Work out the finished part from the listing and answer in its coordinate system (mm). A direction names the side the tool comes from. Give positions to 0.01 mm unless a question says otherwise; leave off trailing zeros. Order: outer loops, then holes, each group sorted by start corner. A loop starts at its lowest first (then second) coordinate and runs counter-clockwise, first axis right, second up. Notation, with made-up numbers: (9, 66.25) - (50, 66.25) arc R23 ccw to (50, 85.25) - close; hole circle Ø11 at (-13, 65.5). An arc over 180 degrees is marked (long way). Put each result on its own line as item: value.
```python
from build123d import *

# Parameters (mm, degrees)
SZKIC1_R                    = 42
DODANIE_WYCI_GNI_CIE1_DEPTH = 200
SFAZOWANIE1_SIZE            = 10
SKORUPA1_T                  = -0.2
SZKIC8_R                    = 32
DODANIE_WYCI_GNI_CIE4_DEPTH = 0.2


with BuildPart() as part:
    # Szkic1 → Dodanie-wyciągnięcie1 (new body)
    with BuildSketch(Plane(origin=(0, 0, 0), x_dir=(1, 0, 0), z_dir=(0, 1, 0))):
        with Locations(Location((0, 0, 0), (0, 0, 270))):
            Circle(SZKIC1_R)
    extrude(amount=DODANIE_WYCI_GNI_CIE1_DEPTH)

    # Sfazowanie1
    sfazowanie1_edges = [part.edges().sort_by_distance(p)[0] for p in [
        (0, 0, -42),
        (0, 200, -42),
    ]]
    chamfer(sfazowanie1_edges, length=SFAZOWANIE1_SIZE)

    # Skorupa1
    skorupa1_openings = [part.faces().sort_by_distance(p)[0] for p in [
        (0, 200, 0),
    ]]
    offset(amount=SKORUPA1_T, openings=skorupa1_openings, kind=Kind.INTERSECTION)

    # Szkic8 → Dodanie-wyciągnięcie4 (add)
    with BuildSketch(Plane(origin=(0, 200, 0), x_dir=(1, 0, 0), z_dir=(0, 1, 0))):
        Circle(SZKIC8_R)
    extrude(amount=-DODANIE_WYCI_GNI_CIE4_DEPTH)


solid = part.part
```
(1) Determine the mould class of faces 1 (the face through (9.76, 199.51, 30.99)), 2 (the face through (-19.71, 0.68, -25.71)), 3 (the face through (0, 199.8, 0)), 4 (the face through (12.62, 98.74, 40.06)) for opening direction Y: pulls with the +Y half, pulls with the -Y half, needs draft (parallel to the pull), parting line crosses it, or undercut.
Geometry check:
face 1: pulls with the +Y half
face 2: undercut
face 3: undercut
face 4: needs draft
(2) A tool of negligible diameter and unlimited length cuts with its end or side. For faces 5 (the face through (9.76, 0.49, 30.99)), 6 (the face through (12.56, 98.74, 39.87)), from which of +Z, -Z, +X, -X, +Y, -Y can it reach the whole face along a straight path? Write none if from no direction.
Geometry check:
face 5: -Y
face 6: none
(3) Straight lines are drawn through the part: line 1 (Y direction, x = 17, z = 14.5); line 2 (X direction, y = 144, z = 0); line 3 (X direction, y = 107, z = -29). For each, find the intervals that lie inside material, in ascending order.
Geometry check:
line 1: y = 0 to 0.2, 199.8 to 200
line 2: x = -42 to -41.8, 41.8 to 42
line 3: x = -30.38 to -30.1, 30.1 to 30.38
(4) Given pin 1 (10 mm diameter, centred on y = 122.5, z = -25.5, fed in from -X); pin 2 (6 mm diameter, centred on y = 68, z = 11.5, fed in from +X); pin 3 (1 mm diameter, centred on y = 178, z = -12, fed in from +X), each flat-ended and moving along its own axis, determine where each tip first touches the part or whether it passes through.
Geometry check:
pin 1: stops at x = -36.66
pin 2: stops at x = 41.13
pin 3: stops at x = 40.39
(5) Section C-C, the plane y = 171.5 is taken. Write down the section's boundary in (x, z).
Geometry check:
outline: circle Ø84 at (0, 0); hole circle Ø83.6 at (0, 0)
(6) Section B-B, the plane x = 0 is taken. Write down the section's boundary in (y, z), then the cut area to 3 significant figures.
Geometry check:
outline: (0, -32) - (10, -42) - (190, -42) - (200, -32) - (200, 32) - (190, 42) - (10, 42) - (0, 32) - close; hole (0.2, -31.92) - (10.08, -41.8) - (189.92, -41.8) - (199.8, -31.92) - (199.8, 31.92) - (189.92, 41.8) - (10.08, 41.8) - (0.2, 31.92) - close
area: 109 mm²
(7) Section A-A, the plane z = 0 is taken. Write down the section's boundary in (x, y).
Geometry check:
outline: (-42, 10) - (-32, 0) - (32, 0) - (42, 10) - (42, 190) - (32, 200) - (-32, 200) - (-42, 190) - close; hole (-41.8, 10.08) - (-31.92, 0.2) - (31.92, 0.2) - (41.8, 10.08) - (41.8, 189.92) - (31.92, 199.8) - (-31.92, 199.8) - (-41.8, 189.92) - close
